from build123d import *

# Parameters (mm, degrees)
BOSS_EXTRUDE1_DEPTH = 5
SKETCH1_4_R         = 0.8
SKETCH1_4_W         = 6
SKETCH1_4_H         = 12.7
BOSS_EXTRUDE3_DEPTH = 1.2
SKETCH4_W           = 8
SKETCH4_H           = 5
BOSS_EXTRUDE5_DEPTH = 2.9


with BuildPart() as part:
    # Sketch1 → Boss-Extrude1 (new body)
    with BuildSketch(Plane(origin=(0, 0, 0), x_dir=(1, 0, 0), z_dir=(0, 1, 0))):
        Polygon((-8.705745229, 33.9), (-8.705745229, 35.7), (-2.705745229, 35.7), (-2.705745229, 33.9), (-2.705745229, 21.2), (-8.705745229, 21.2), align=None)
    extrude(amount=BOSS_EXTRUDE1_DEPTH)

    # Sketch1_4 → Boss-Extrude3 (add)
    # profile 1 of 2: a face of its own
    with BuildSketch(Plane(origin=(0, 0, 0), x_dir=(1, 0, 0), z_dir=(0, 1, 0))):
        with BuildLine():
            Line((-8.705745229, 21.2), (-8.705745229, 33.9))
            ThreePointArc((-8.705745229, 33.9), (0, -35), (8.705745229, 33.9))
            Line((8.705745229, 33.9), (3.894254771, 33.9))
            Line((3.894254771, 33.9), (-2.705745229, 33.9))
            Line((-2.705745229, 33.9), (-2.705745229, 21.2))
            Line((-2.705745229, 21.2), (-8.705745229, 21.2))
        make_face()
        with Locations(Location((7.14, -28, 0), (0, 0, 270))):
            Circle(SKETCH1_4_R, mode=Mode.SUBTRACT)
        with Locations(Location((-18.963757819, 11.9, 0), (0, 0, 270))):
            Circle(SKETCH1_4_R, mode=Mode.SUBTRACT)
        with Locations(Location((18.963757819, 11.9, 0), (0, 0, 270))):
            Circle(SKETCH1_4_R, mode=Mode.SUBTRACT)
    # profile 2 of 2: a face of its own
    with BuildSketch(Plane(origin=(0, 0, 0), x_dir=(1, 0, 0), z_dir=(0, 1, 0))):
        with Locations((-5.705745229, 27.55)):
            Rectangle(SKETCH1_4_W, SKETCH1_4_H)
    extrude(amount=-BOSS_EXTRUDE3_DEPTH)

    # Sketch4 → Boss-Extrude5 (add)
    with BuildSketch(Plane(origin=(0, 0, 0), x_dir=(1, 0, 0), z_dir=(0, 1, 0))):
        with Locations((7.294254771, 31.4)):
            Rectangle(SKETCH4_W, SKETCH4_H)
    extrude(amount=BOSS_EXTRUDE5_DEPTH)


solid = part.part
Can you work these out from the model? Positions are in its coordinate system, mm. A direction names the side the tool comes from. Coordinates: 2 decimals unless noted, no trailing zeros. Order: outer loops, then holes, each group sorted by start corner. A loop starts at its lowest first (then second) coordinate and runs counter-clockwise, first axis right, second up. Notation, with made-up numbers: (38, 5.25) - (42, 5.25) arc R22 ccw to (42, 44.25) - close; hole circle Ø11 at (87, -18). An arc over 180 degrees is marked (long way). Answer as a JSON object with one key per item and string values. Group by question number.
Q1. Imagine slicing it at C-C (x = -5). Please give me the cut outline in (y, z).
Q2. Imagine slicing it at D-D (z = -11.9). Please give me the cut outline in (x, y).
Q3. Imagine slicing it at A-A (z = 28). Please give me the cut outline in (x, y), and give its area (3 significant figures).
Q4. Will these pins go through, and if not, where does the flat tip stop? P1, Ø2.5, axis at y = 1.5, z = -28, coming from the +X side; P2, Ø5, axis at x = -17, z = 6, coming from the +Y side; P3, Ø1.5, axis at y = 1.5, z = -27.5, coming from the -X side; P4, Ø1, axis at x = 7.14, z = 28, coming from the +Y side.
Q5. Imagine slicing it at B-B (x = 7.14). Please give me the cut outline in (y, z), and give its area (3 significant figures).
Q6. On a 3-axis mill with a long thin cutter (end or side, diameter ignored), from which of +Z, -Z, +X, -X, +Y, -Y can I reach the whole of each face in a straight line? I mean faces 4 (the face through (-6, 2, -21.2)), 5 (the face through (-8.706, 2, -29)), 6 (the face through (3, -1, -33.9)). Say none if no direction works.
Q7. I need wall thicknesses on line 1 (X direction, y = -0.9, z = -11.9); line 2 (Y direction, x = 23.5, z = -11.5); line 3 (Z direction, x = -5, y = 1.5). Which ranges of each line are inside material? Lowest first, please. Write a range as from..to.
Q8. We'd pull the mould along X, two halves only. Please class faces 1 (the face through (-19.673, -0.592, -11.531)), 2 (the face through (-6, 0, -35)), 3 (the face through (-1.42, -0.59, 34.97)): +X half, -X half, draft (parallel to the pull), parting line (faces both ways), or undercut.
Determined:
{
 "1": {"outline": "(-1.2, -33.9) - (0, -33.9) - (0, -35.7) - (5, -35.7) - (5, -21.2) - (0, -21.2) - (0, 34.64) - (-1.2, 34.64) - close"},
 "2": {"outline": "(-32.91, -1.2) - (-19.76, -1.2) - (-19.76, 0) - (-32.91, 0) - close; (-18.16, -1.2) - (18.16, -1.2) - (18.16, 0) - (-18.16, 0) - close; (19.76, -1.2) - (32.91, -1.2) - (32.91, 0) - (19.76, 0) - close"},
 "3": {"outline": "(-21, -1.2) - (6.34, -1.2) - (6.34, 0) - (-21, 0) - close; (7.94, -1.2) - (21, -1.2) - (21, 0) - (7.94, 0) - close", "area": "48.5 mm2"},
 "4": {"P1": "stops at x = 11.29", "P2": "stops at y = 0", "P3": "stops at x = -8.71", "P4": "passes through"},
 "5": {"outline": "(-1.2, -33.9) - (2.9, -33.9) - (2.9, -28.9) - (0, -28.9) - (0, 27.2) - (-1.2, 27.2) - close; (-1.2, 28.8) - (0, 28.8) - (0, 34.26) - (-1.2, 34.26) - close", "area": "94.4 mm2"},
 "6": {"face 4": "+Z, +X, -X, +Y", "face 5": "+Z, -Z, -X, +Y", "face 6": "-Z, +X, -Y"},
 "7": {"line 1": "x = -32.91..-19.76, -18.16..18.16, 19.76..32.91", "line 2": "y = -1.2..0", "line 3": "z = -35.7..-21.2"},
 "8": {"face 1": "undercut", "face 2": "draft", "face 3": "parting line"}
}
